Read the model definition and answer for the solid it produces. Units are mm, in the model's axes. Face numbers are marked on the shaded views. A direction names the side the tool comes from. Coordinates: 2 decimals unless noted, no trailing zeros. Order: outer loops, then holes, each group sorted by start corner. A loop starts at its lowest first (then second) coordinate and runs counter-clockwise, first axis right, second up. Notation, with made-up numbers: M 20,-15 L 43,-15 A25 ccw 43,6 Z; hole C 14,31.25 d1. An arc over 180 degrees is marked long. Put each result on its own line as item: value.
from build123d import *

# Parameters (mm, degrees)
F1_DEPTH = 60
F2_R     = 2.6
F3_DEPTH = 25.001
F6_DEPTH = 25
F7_W     = 8
F7_H     = 8
F8_DEPTH = 60.0010001


with BuildPart() as f1:
    # F0 (on Top) → F1 (new body)
    with BuildSketch(Plane.XY):
        with BuildLine():
            Line((0, -14), (0, -25))
            ThreePointArc((0, -25), (25, 0), (0, 25))
            Line((0, 25), (0, 14))
            ThreePointArc((0, 14), (14, 0), (0, -14))
        make_face()
    extrude(amount=F1_DEPTH)

    # F2 (on Right) → F3 (cut, through all)
    with BuildSketch(Plane.YZ):
        with Locations((-20.5, 10)):
            Circle(F2_R)
        with Locations((-20.5, 50)):
            Circle(F2_R)
        with Locations((20.5, 50)):
            Circle(F2_R)
        with Locations((20.5, 10)):
            Circle(F2_R)
    extrude(amount=F3_DEPTH, mode=Mode.SUBTRACT)

    # F5 (on offset) → F6 (cut)
    with BuildSketch(Plane(origin=(6, 0, 0), x_dir=(0, -1, 0), z_dir=(-1, 0, 0))):
        with BuildLine():
            ThreePointArc((15.25, 50), (20.5, 44.75), (25.75, 50))
            ThreePointArc((25.75, 50), (20.5, 55.25), (15.25, 50))
        make_face()
        with BuildLine():
            ThreePointArc((-15.25, 10), (-16.7876893988, 13.7123106012), (-20.5, 15.25))
            ThreePointArc((-20.5, 15.25), (-24.2123106012, 6.2876893988), (-15.25, 10))
        make_face()
    extrude(amount=-F6_DEPTH, mode=Mode.SUBTRACT)

    # F7 (on Top) → F8 (cut, through all)
    with BuildSketch(Plane.XY):
        with Locations((16, 0)):
            Rectangle(F7_W, F7_H)
    extrude(amount=F8_DEPTH, mode=Mode.SUBTRACT)


solid = f1.part
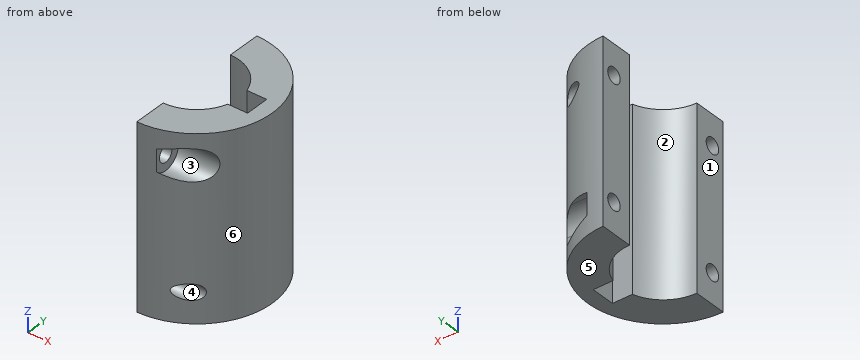
Q1. Consider line 1 along Z through (x, y) = (9.5, -20.5); line 2 along Z through (x, y) = (1.5, 20.5); line 3 along Y through (x, z) = (9, 50). Determine where each line is inside the solid, lowest interval first.
Answers below:
line 1: z = 0 to 7.4, 12.6 to 44.75, 55.25 to 60
line 2: z = 0 to 7.4, 12.6 to 47.4, 52.6 to 60
line 3: y = -15.25 to -10.72, 10.72 to 17.9, 23.1 to 23.32
Q2. Find section B-B on x = 3.75. Write down the section's boundary in (y, z), plus the area to 3 significant figures.
Answers below:
outline: M -24.72,0 L -13.49,0 L -13.49,60 L -24.72,60 Z; M 13.49,0 L 24.72,0 L 24.72,60 L 13.49,60 Z; hole C -20.5,10 d5.2; hole C -20.5,50 d5.2; hole C 20.5,10 d5.2; hole C 20.5,50 d5.2
area: 1,260 mm^2
Q3. For a pull along Y with two mould halves and no side action, classify the marked faces 4, 5 and 6 as +Y half, -Y half, draft (parallel to the pull), parting line (faces both ways), or undercut.
Answers below:
face 4: undercut
face 5: draft
face 6: parting line
Q4. Find section D-D on z = 22.5. Write down the section's boundary in (x, y), plus the area to 3 significant figures.
Answers below:
outline: M 0,-25 A25 ccw 0,25 L 0,14 A14 cw 13.42,4 L 20,4 L 20,-4 L 13.42,-4 A14 cw 0,-14 Z
area: 624 mm^2
Q5. Given pin 1 (2 mm diameter, centred on x = 17.5, z = 34, fed in from +Y); pin 2 (1.5 mm diameter, centred on y = -12, z = 14, fed in from -X); pin 3 (10 mm diameter, centred on y = 20.5, z = 12, fed in from +X); pin 4 (6.5 mm diameter, centred on y = -20.5, z = 50, fed in from -X), each flat-ended and moving along its own axis, determine where each tip first touches the part or whether it passes through.
Answers below:
pin 1: stops at y = 18.78
pin 2: stops at x = 5.78
pin 3: stops at x = 19.62
pin 4: stops at x = 0
Q6. Find section A-A on y = -20.5. Write down the section's boundary in (x, z).
Answers below:
outline: M 0,0 L 14.31,0 L 14.31,7.4 L 0,7.4 Z; M 0,12.6 L 14.31,12.6 L 14.31,44.75 L 6,44.75 L 6,47.4 L 0,47.4 Z; M 0,52.6 L 6,52.6 L 6,55.25 L 14.31,55.25 L 14.31,60 L 0,60 Z
Q7. A tool of negligible diameter and unlimited length cuts with its end or side. For the marked faces 1, 2 and 3, from which of +Z, -Z, +X, -X, +Y, -Y can it reach the whole face along a straight path? Write none if from no direction.
Answers below:
face 1: +Z, -Z, -X, +Y, -Y
face 2: +Z, -Z, -X
face 3: +X
Q8. Find section C-C on x = 11.25. Write down the section's boundary in (y, z), plus the area to 3 significant figures.
Answers below:
outline: M -22.33,0 L -8.33,0 L -8.33,60 L -22.33,60 L -22.33,54.92 A5.25 cw long -22.33,45.08 L -22.33,11.85 A2.6 cw long -22.33,8.15 Z; M 8.33,0 L 22.33,0 L 22.33,5.08 A5.25 cw long 22.33,14.92 L 22.33,48.15 A2.6 cw long 22.33,51.85 L 22.33,60 L 8.33,60 Z
area: 1,520 mm^2
